Here's how the part is built. I have some questions about the finished solid (model axes, mm). A direction names the side the tool comes from. Round coordinates to 2 decimals unless told otherwise and drop trailing zeros. Write each loop counter-clockwise with the first axis right and the second up, starting at its lowest first coordinate (ties: lowest second). Pieces come first, ordered by that corner, then holes. Notation, with made-up numbers: M 28.25,61 L 47.25,61 A31 cw 47.25,96 Z; hole C 76,6.25 d4. An arc over 180 degrees is marked long. Write item = value, one per line. Start each with the question number.
(1) I need wall thicknesses on line 1 along Z through (x, y) = (42.5, 2.15) (1 decimal); line 2 along Y through (x, z) = (94, 35.5). Which ranges of each line are inside material? Lowest first, please.
(2) I want a section at A-A (y = 2.6). List the corners of the cut face in (x, z) for me (1 decimal).
(3) On a 3-axis mill with a long thin cutter (end or side, diameter ignored), from which of +Z, -Z, +X, -X, +Y, -Y can I reach the whole of each face in a straight line? I mean faces 4 (the flat face through (53, 0, 19)), 5 (the flat face through (52, 1.588, 5)). Say none if no direction works.
(4) Will this pin go through, and if not, where does the flat tip stop? pin 1 Ø1 at (x, z) = (41.5, 5) entering from +Y.
(5) I want a section at B-B (x = 63.5). List the corners of the cut face in (y, z) for me (1 decimal), and give its area (3 significant figures).
(6) If we mould it in two halves opening along X, with no side actions, what happens to faces 1 (the flat face through (0, 2, 19)), 2 (the flat face through (53, 3.175, 20)), 3 (the flat face through (104.775, 2, 19))? For each: released by +X, released by -X, zero draft, split by the parting line, or undercut.
(7) I want a section at C-C (z = 35.5). List the corners of the cut face in (x, y) for me (1 decimal).
Autodesk Inventor part; units mm, degrees
ref_plane "YZ Plane" through (0, 0, 0) normal (1, 0, 0) x (0, 1, 0)
ref_plane "XZ Plane" through (0, 0, 0) normal (0, 1, 0) x (-1, 0, 0)
ref_plane "XY Plane" through (0, 0, 0) normal (0, 0, 1) x (1, 0, 0)
sketch "Sketch1" plane through (0, 0, 0) normal (0, 1, 0) x (-1, 0, 0)
  line L0 (0, 0) -> (-104.775, 0)
  line L1 (-104.775, 0) -> (-104.775, 38.1)
  line L2 (-104.775, 38.1) -> (0, 38.1)
  line L3 (0, 38.1) -> (0, 0)
  dimension "d0" = 104.775
  dimension "d1" = 38.1
extrude "Extrusion1" add sketch "Sketch1" along normal blind 3.175
sketch "Sketch2" plane through (0, 3.175, 0) normal (0, 1, 0) x (1, 0, 0)
  line L0 (0, 0) -> (0, -38.1)
  line L1 (104.775, -38.1) -> (104.775, 0)
  line L2 (0, -33.3121) -> (104.775, -33.3121)
  line L3 (104.775, -33.3121) -> (104.775, -36.5125)
  line L4 (104.775, -36.5125) -> (0, -36.5125)
  line L5 (0, -36.5125) -> (0, -33.3121)
  line L6 (0, -38.1) -> (104.775, -38.1)
  line L7 (104.775, 0) -> (0, 0)
  line L8 (104.775, -3.175) -> (0, -3.175)
  line L9 (0, -3.175) -> (0, -6.604)
  line L10 (0, -6.604) -> (104.775, -6.604)
  line L11 (104.775, -6.604) -> (104.775, -3.175)
  dimension "d4" = 3.2004
  dimension "d8" = 1.5875
  dimension "d13" = 3.175
  dimension "d14" = 3.429
extrude "Extrusion2" cut sketch "Sketch2" against normal blind 1.5875 contours L8 L1 L10 L0 | L2 L1 L4 L0
properties part number "Electronics Container Part 2"
Returned:
q1.line_1 = 0 to 3.2, 6.6 to 33.3, 36.5 to 38.1
q1.line_2 = 0 to 1.59
q2.outline = M 0,0 L 104.8,0 L 104.8,3.2 L 0,3.2 Z; M 0,6.6 L 104.8,6.6 L 104.8,33.3 L 0,33.3 Z; M 0,36.5 L 104.8,36.5 L 104.8,38.1 L 0,38.1 Z
q3.face_4 = +Z, -Z, +X, -X, -Y
q3.face_5 = +X, -X, +Y
q4.pin_1 = 1.59
q5.outline = M 0,0 L 3.2,0 L 3.2,3.2 L 1.6,3.2 L 1.6,6.6 L 3.2,6.6 L 3.2,33.3 L 1.6,33.3 L 1.6,36.5 L 3.2,36.5 L 3.2,38.1 L 0,38.1 Z
q5.area = 110 mm²
q6.face_1 = released by -X
q6.face_2 = zero draft
q6.face_3 = released by +X
q7.outline = M 0,0 L 104.8,0 L 104.8,1.6 L 0,1.6 Z
